For this review, take the finished solid that the model builds, in its own axes (mm). Coordinates: 2 decimals unless noted, no trailing zeros. Order: outer loops, then holes, each group sorted by start corner. A loop starts at its lowest first (then second) coordinate and runs counter-clockwise, first axis right, second up.
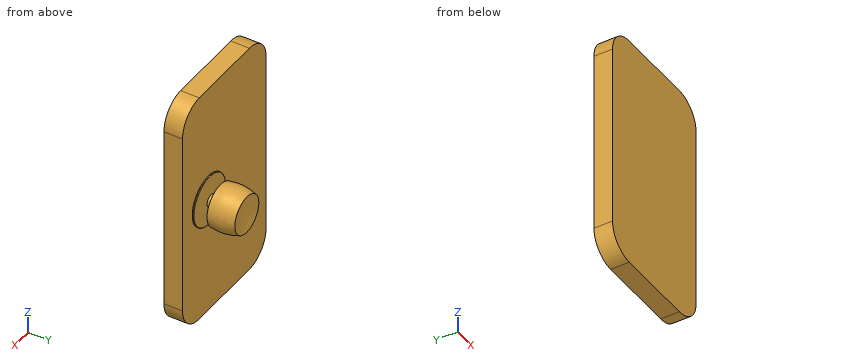
from build123d import *

# Parameters (mm, degrees)
SKETCH1_W           = 127
SKETCH1_H           = 228.6
BOSS_EXTRUDE1_DEPTH = 17.78
FILLET1_R           = 25.4


with BuildPart() as part:
    # Sketch1 → Boss-Extrude1 (new body)
    with BuildSketch(Plane(origin=(0, 0, 0), x_dir=(1, 0, 0), z_dir=(0, 1, 0))):
        Rectangle(SKETCH1_W, SKETCH1_H)
    extrude(amount=BOSS_EXTRUDE1_DEPTH)

    # Fillet1
    fillet1_edges = [part.edges().sort_by_distance(p)[0] for p in [
        (63.5, 8.89, 114.3),
        (-63.5, 8.89, 114.3),
        (-63.5, 8.89, -114.3),
        (63.5, 8.89, -114.3),
    ]]
    fillet(fillet1_edges, radius=FILLET1_R)

    # Sketch3 → Revolve1 (revolve)
    with BuildSketch(Plane.XY):
        with BuildLine():
            Line((24.400711068, 17.78), (0, 17.78))
            Line((0, 17.78), (0, 18.621092674))
            ThreePointArc((0, 18.621092674), (0.153192874, 18.984652715), (0.520377573, 19.12894186))
            ThreePointArc((0.520377573, 19.12894186), (9.452590015, 19.351960716), (18.319397174, 20.453726269))
            Line((18.319397174, 20.453726269), (18.319397174, 23.831447825))
            Line((18.319397174, 23.831447825), (18.319397174, 27.940464373))
            Line((18.319397174, 27.940464373), (24.400711068, 27.940464373))
            Line((24.400711068, 27.940464373), (24.400711068, 23.831447825))
            Line((24.400711068, 23.831447825), (24.400711068, 21.732479509))
            Line((24.400711068, 21.732479509), (24.400711068, 17.78))
        make_face()
    revolve(axis=Axis((24.400711068, 21.732479509, 0), (0, -1, 0)))

    # Sketch4 → Revolve2 (revolve)
    with BuildSketch(Plane.XY):
        with BuildLine():
            Line((24.400711068, 27.940464373), (24.400711068, 52.102517499))
            ThreePointArc((24.400711068, 52.102517499), (33.609505059, 52.688947823), (42.630480882, 54.630025491))
            ThreePointArc((42.630480882, 54.630025491), (45.38750409, 42.105790986), (44.646315408, 29.303124613))
            ThreePointArc((44.646315408, 29.303124613), (34.587150849, 27.67630429), (24.400711068, 27.940464373))
        make_face()
    revolve(axis=Axis((24.400711068, 27.940464373, 0), (0, 1, 0)))


solid = part.part
1. To check wall thickness, follow L1, parallel to Y at x = -47.5, z = 39.5; L2, parallel to Z at x = 5.5, y = 45; L3, parallel to Z at x = -46.5, y = 14. State the ranges of each line that lie inside material, in increasing order.
Answer below:
L1: y = 0 to 17.78
L2: z = -8.36 to 8.36
L3: z = -112.87 to 112.87
2. Clearance check with flat-ended pins moving along their axes: pin 1 Ø10 at (x, z) = (-9.5, -61.5) entering from +Y; pin 2 Ø8 at (x, y) = (15.5, 26.5) entering from -Z; pin 3 Ø1 at (y, z) = (19, 17.5) entering from -X. State where each tip first meets the part, or that it passes through.
Answer below:
pin 1: stops at y = 17.78
pin 2: stops at z = -19.32
pin 3: stops at x = 6.98
3. Take a section at A-A, the plane y = 12. Give the boundary of the cut face in (x, z).
Answer below:
outline: (-63.5, -88.9) arc R25.4 ccw to (-38.1, -114.3) - (38.1, -114.3) arc R25.4 ccw to (63.5, -88.9) - (63.5, 88.9) arc R25.4 ccw to (38.1, 114.3) - (-38.1, 114.3) arc R25.4 ccw to (-63.5, 88.9) - close
4. Take a section at B-B, the plane z = 60.5. Give the boundary of the cut face in (x, y), plus the area to 3 significant figures.
Answer below:
outline: (-63.5, 0) - (63.5, 0) - (63.5, 17.78) - (-63.5, 17.78) - close
area: 2,260 mm2
5. Take a section at C-C, the plane x = -11. Give the boundary of the cut face in (y, z).
Answer below:
outline: (0, -114.3) - (17.78, -114.3) - (17.78, 114.3) - (0, 114.3) - close
